Study the drawing (mm; zero at the part's minimum x, y, z) and answer. A direction names the side the tool comes from. Round coordinates to 2 decimals unless told otherwise and drop trailing zeros. Loops run counter-clockwise (first coordinate to the right, second up) from the corner with the lowest first, then second, coordinate; pieces in that order, holes last. Notation, with made-up numbers: (87.5, -3) -> (128.5, -3) arc R16 ccw to (128.5, 20) -> close; hole circle Ø11 at (50, 79). An arc over 180 degrees is marked (long way). Use one line per item in the form item = value.
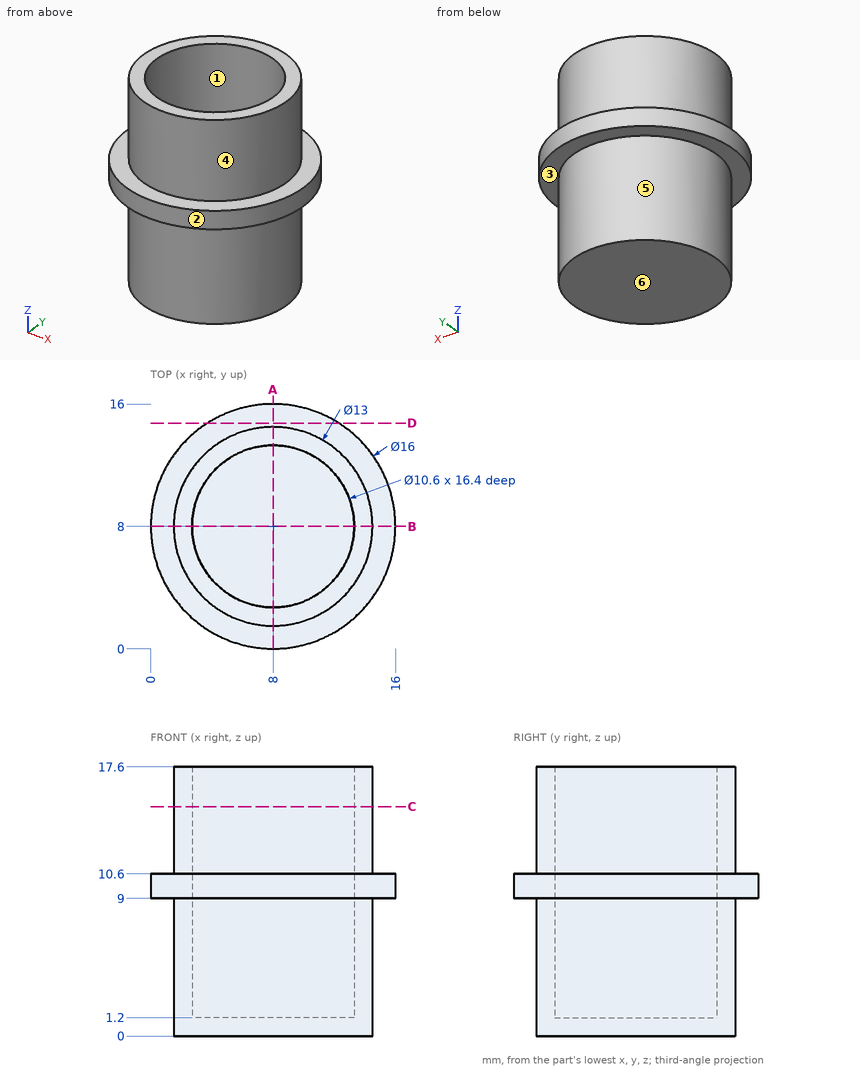
(1) Consider L1, parallel to Y at x = 8, z = 13.75; L2, parallel to Y at x = 8, z = 9.5; L3, parallel to Z at x = 7, y = 8. Determine where each line is inside the solid, lowest interval first.
Completed:
L1 = 1.5 to 2.7, 13.3 to 14.5
L2 = 0 to 2.7, 13.3 to 16
L3 = 0 to 1.2
(2) Find section D-D, the plane y = 14.75. Write down the section's boundary in (x, z), then the cut area to 3 significant figures.
Completed:
outline = (3.71, 9) -> (12.29, 9) -> (12.29, 10.6) -> (3.71, 10.6) -> close
area = 13.7 mm2
(3) Find section C-C, the plane z = 15. Write down the section's boundary in (x, y), then the cut area to 3 significant figures.
Completed:
outline = circle Ø13 at (8, 8); hole circle Ø10.6 at (8, 8)
area = 44.5 mm2
(4) For the marked faces 4, 5 and 6, determine the directions among +Z, -Z, +X, -X, +Y, -Y from which every point of the face is accessible in a straight line to the end or side of a thin tool.
Completed:
face_4 = +Z
face_5 = -Z
face_6 = -Z, +X, -X, +Y, -Y
(5) Find section A-A, the plane x = 8. Write down the section's boundary in (y, z).
Completed:
outline = (0, 9) -> (1.5, 9) -> (1.5, 0) -> (14.5, 0) -> (14.5, 9) -> (16, 9) -> (16, 10.6) -> (14.5, 10.6) -> (14.5, 17.6) -> (13.3, 17.6) -> (13.3, 1.2) -> (2.7, 1.2) -> (2.7, 17.6) -> (1.5, 17.6) -> (1.5, 10.6) -> (0, 10.6) -> close
(6) For a pull along Y with two mould halves and no side action, classify the marked faces 1, 2 and 3 as +Y half, -Y half, draft (parallel to the pull), parting line (faces both ways), or undercut.
Completed:
face_1 = undercut
face_2 = parting line
face_3 = draft
(7) Given P1, Ø3, axis at x = 2, z = 13, coming from the +Y side; P2, Ø8, axis at x = 11.5, z = 8.5, coming from the -Y side; P3, Ø3, axis at x = 8.5, y = 6, coming from the +Z side; P4, Ø5, axis at y = 5.5, z = 7.5, coming from the -X side, each flat-ended and moving along its own axis, determine where each tip first touches the part or whether it passes through.
Completed:
P1 = 12.69
P2 = 0
P3 = 1.2
P4 = 0.02
